Design review of the part shown in the three views and the two pictorial views. Dimensions are in mm from the part's minimum x, y and z. A direction names the side the tool comes from. Round coordinates to 2 decimals unless told otherwise and drop trailing zeros. Order: outer loops, then holes, each group sorted by start corner. A loop starts at its lowest first (then second) coordinate and runs counter-clockwise, first axis right, second up.
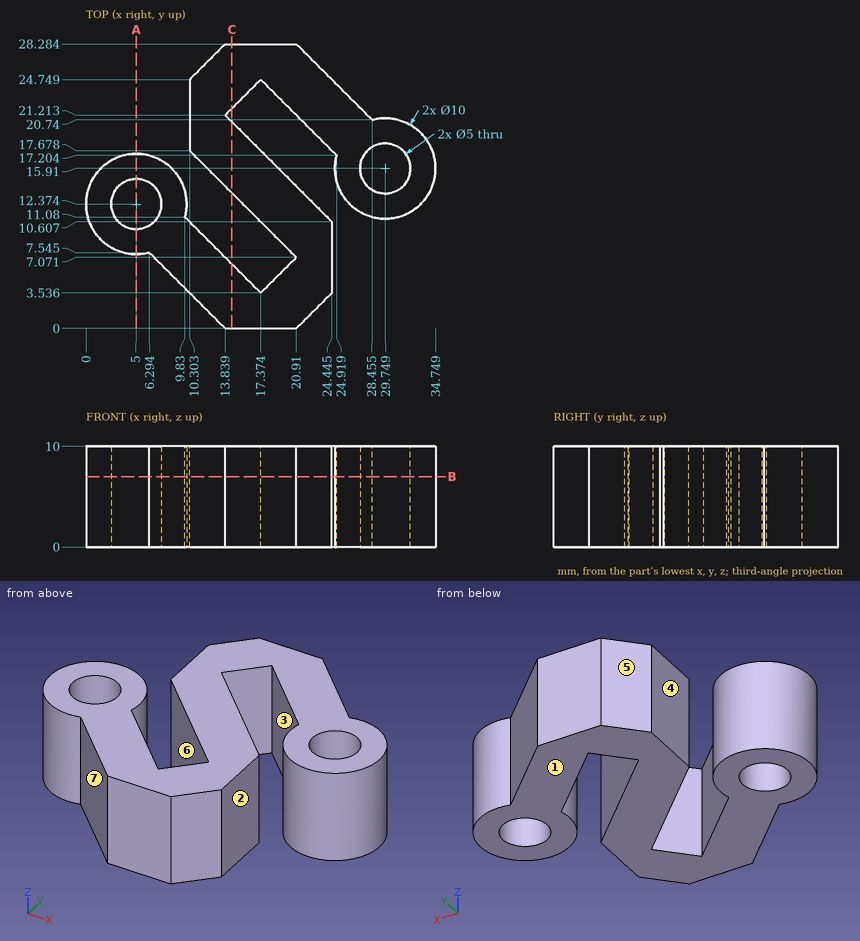
(1) Tool access review of the marked faces 1, 2, 3 and 4: name each direction out of +Z, -Z, +X, -X, +Y, -Y from which nothing blocks a thin tool from reaching the whole face with its end or side.
(2) Draft analysis for pull direction Y (two halves, no side actions). For the marked faces 5, 6 and 7, state which applies: pulls with the +Y half, pulls with the -Y half, needs draft (parallel to the pull), parting line crosses it, or undercut.
(3) Clearance check with flat-ended pins moving along their axes: P1, Ø3, axis at x = 9, z = 9, coming from the -Y side; P2, Ø4, axis at y = 18.5, z = 2.5, coming from the -X side (1 decimal); P3, Ø3, axis at y = 11.5, z = 6, coming from the +X side (1 decimal). State where each tip first meets the part, or that it passes through.
(4) Add section A-A on x = 5. Give the boundary of the cut face in (y, z) (1 decimal).
(5) Wall thickness on L1, parallel to Y at x = 5, z = 6.25 (1 decimal); L2, parallel to X at y = 3.75, z = 9.75 (1 decimal); L3, parallel to Y at x = 3, z = 9 (1 decimal): over which ranges is each line inside the solid? List them lowest first.
(6) Add section C-C on x = 14.5. Give the boundary of the cut face in (y, z) (1 decimal).
(7) Add section B-B on z = 7. Give the boundary of the cut face in (x, y) (1 decimal).
Here are the results:
1. face 1: -Z, +X, -X, +Y, -Y
1. face 2: +Z, -Z, +X, -Y
1. face 3: +Z, -Z
1. face 4: +Z, -Z, -X, +Y
2. face 5: pulls with the +Y half
2. face 6: undercut
2. face 7: pulls with the -Y half
3. P1: stops at y = 3.34
3. P2: stops at x = 2.2
3. P3: stops at x = 33.8
4. outline: (7.4, 0) - (9.9, 0) - (9.9, 10) - (7.4, 10) - close; (14.9, 0) - (17.4, 0) - (17.4, 10) - (14.9, 10) - close
5. L1: y = 7.4 to 9.9, 14.9 to 17.4
5. L2: x = 10.1 to 17.2, 17.6 to 24.4
5. L3: y = 7.8 to 10.9, 13.9 to 17
6. outline: (0, 0) - (6.4, 0) - (6.4, 10) - (0, 10) - close; (13.5, 0) - (20.6, 0) - (20.6, 10) - (13.5, 10) - close; (21.9, 0) - (28.3, 0) - (28.3, 10) - (21.9, 10) - close
7. outline: (6.3, 7.5) - (13.8, 0) - (20.9, 0) - (24.4, 3.5) - (24.4, 10.6) - (13.8, 21.2) - (17.4, 24.7) - (24.9, 17.2) arc R5 ccw (long way) to (28.5, 20.7) - (20.9, 28.3) - (13.8, 28.3) - (10.3, 24.7) - (10.3, 17.7) - (20.9, 7.1) - (17.4, 3.5) - (9.8, 11.1) arc R5 ccw (long way) to start; hole circle Ø5 at (5, 12.4); hole circle Ø5 at (29.7, 15.9)
